Here's the drawing with two shaded views (mm, measured from the low corner). I have some questions. Coordinates: 2 decimals unless noted, no trailing zeros. Write each loop counter-clockwise with the first axis right and the second up, starting at its lowest first coordinate (ties: lowest second). Pieces come first, ordered by that corner, then holes. Notation, with made-up numbers: (10.5, 57) -> (25.5, 57) arc R11 ccw to (25.5, 61) -> close; hole circle Ø10 at (9, -12.5). An arc over 180 degrees is marked (long way). Use one line per item in the form item = value.
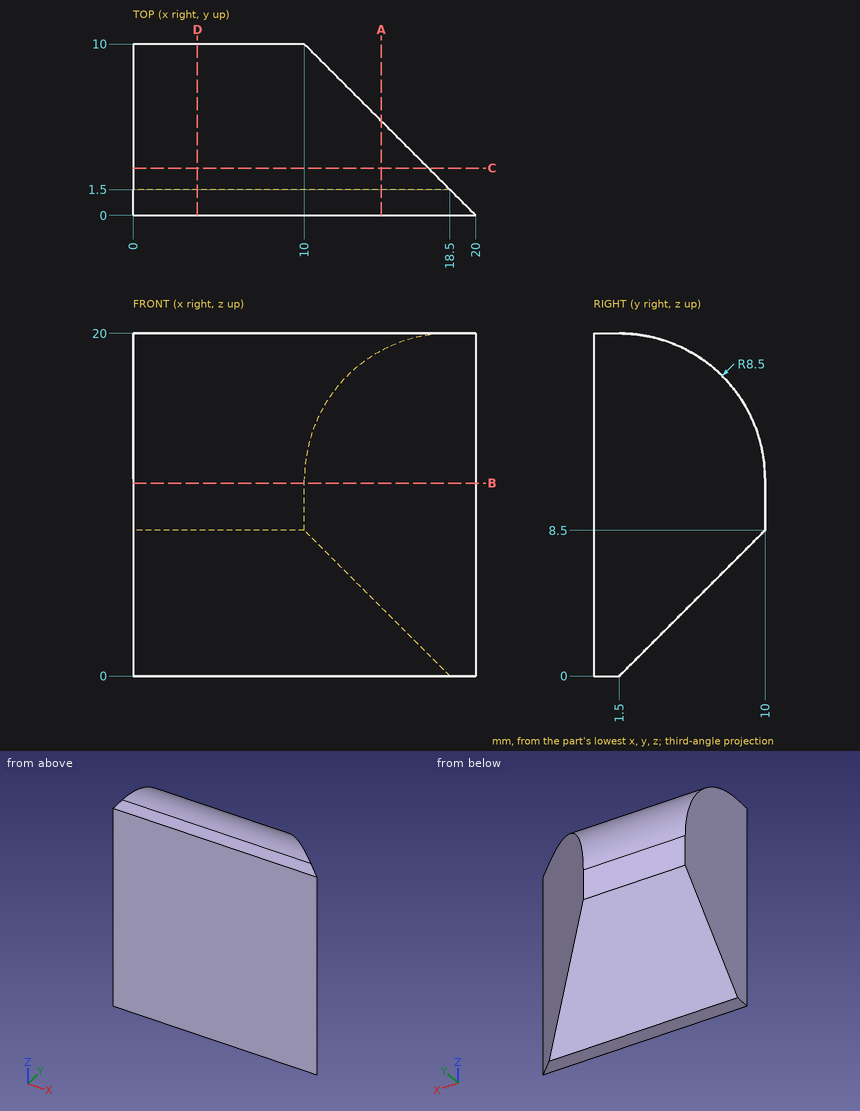
Q1. Suppose I cut it at A-A (x = 14.5). Write out the boundary of the cut face in (y, z), then the cut area to 3 significant figures.
Return value:
outline = (0, 0) -> (1.5, 0) -> (5.5, 4) -> (5.5, 19) arc R8.5 ccw to (1.5, 20) -> (0, 20) -> close
area = 101 mm2
Q2. Suppose I cut it at B-B (z = 11.25). Write out the boundary of the cut face in (x, y), then the cut area to 3 significant figures.
Return value:
outline = (0, 0) -> (20, 0) -> (10, 10) -> (0, 10) -> close
area = 150 mm2
Q3. Suppose I cut it at D-D (x = 3.75). Write out the boundary of the cut face in (y, z), then the cut area to 3 significant figures.
Return value:
outline = (0, 0) -> (1.5, 0) -> (10, 8.5) -> (10, 11.5) arc R8.5 ccw to (1.5, 20) -> (0, 20) -> close
area = 148 mm2
Q4. Will these pins go through, and if not, where does the flat tip stop? pin 1 (2 mm diameter, centred on x = 15.5, y = 5.5, fed in from -Z); pin 2 (5 mm diameter, centred on y = 4.5, z = 17, fed in from +X); pin 3 (1.5 mm diameter, centred on x = 5, z = 16.5, fed in from +Y).
Return value:
pin_1 = 3
pin_2 = 18
pin_3 = 8.86
Q5. Suppose I cut it at C-C (y = 2.75). Write out the boundary of the cut face in (x, z), then the cut area to 3 significant figures.
Return value:
outline = (0, 1.25) -> (17.25, 1.25) -> (17.25, 19.91) -> (0, 19.91) -> close
area = 322 mm2
Q6. If I drill on line 1 (Y direction, x = 18.5, z = 10.25); line 2 (Y direction, x = 10, z = 12); line 3 (X direction, y = 6.25, z = 12), over which ranges is the centre line in solid material (lowest first)? Write a range as from..to.
Return value:
line_1 = 0..1.5
line_2 = 0..9.99
line_3 = 0..13.75
